The model under review builds one solid part; all positions refer to its coordinate system, in mm. Face numbers are marked on the shaded views. A direction names the side the tool comes from. Give positions to 0.01 mm unless a question says otherwise; leave off trailing zeros. Order: outer loops, then holes, each group sorted by start corner. A loop starts at its lowest first (then second) coordinate and runs counter-clockwise, first axis right, second up. Notation, with made-up numbers: (10, 63) - (59, 63) arc R17 cw to (59, 94) - close; hole circle Ø5 at (25, -12). An arc over 180 degrees is marked (long way). Use CSV: the item, a comma, the result in double quotes.
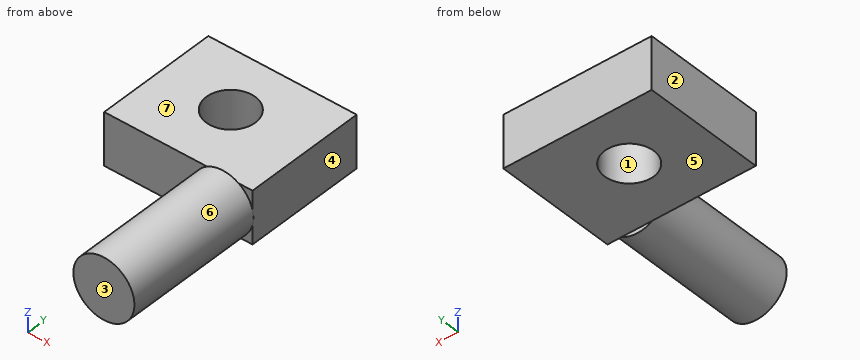
Autodesk Inventor part; units mm, degrees
ref_plane "YZ Plane" through (0, 0, 0) normal (1, 0, 0) x (0, 1, 0)
ref_plane "XZ Plane" through (0, 0, 0) normal (0, 1, 0) x (-1, 0, 0)
ref_plane "XY Plane" through (0, 0, 0) normal (0, 0, 1) x (1, 0, 0)
sketch "Sketch1" plane through (0, 0, 0) normal (0, 1, 0) x (-1, 0, 0)
  circle A0 centre (0, 0) radius 17.5
  dimension "d0" = 35
extrude "Extrusion1" add sketch "Sketch1" along normal blind 80
sketch "Sketch2" plane through (0, 80, 0) normal (0, 1, 0) x (1, 0, 0)
  line L0 (-68, -15) -> (17, -15)
  line L1 (17, -15) -> (17, 15)
  line L2 (17, 15) -> (-68, 15)
  line L3 (-68, 15) -> (-68, -15)
  point P0 (0, 0)
  dimension "d3" = 85
  dimension "d4" = 30
extrude "Extrusion2" add sketch "Sketch2" along normal blind 70
sketch "Sketch3" plane through (-68, 80, 15) normal (0, 0, 1) x (1, 0, 0)
  circle A0 centre (41, 37) radius 14
  point P0 (68, -80)
extrude "Extrusion3" cut sketch "Sketch3" against normal through all
properties part number "motor hombro"
Item 1: Wall thickness on L1, parallel to Y at x = -27, z = 6; L2, parallel to Z at x = -60.5, y = 123; L3, parallel to Y at x = -48, z = -2.5: over which ranges is each line inside the solid? List them lowest first.
Results list:
L1,"y = 80 to 103, 131 to 150"
L2,"z = -15 to 15"
L3,"y = 80 to 150"
Item 2: Take a section at B-B, the plane z = 0. Give the boundary of the cut face in (x, y), and give its area (3 significant figures).
Results list:
outline,"(-68, 80) - (-17.5, 80) - (-17.5, 0) - (17.5, 0) - (17.5, 80) - (17, 80) - (17, 150) - (-68, 150) - close; hole circle Ø28 at (-27, 117)"
area,"8,130 mm2"
Item 3: Mouldability with a two-part tool opening along X and no side actions: class the marked faces 1, 2, 3 and 4 as pulls with the +X half, pulls with the -X half, needs draft (parallel to the pull), parting line crosses it, or undercut.
Results list:
face 1,"undercut"
face 2,"pulls with the -X half"
face 3,"needs draft"
face 4,"pulls with the +X half"
Item 4: Take a section at C-C, the plane x = -31. Give the boundary of the cut face in (y, z).
Results list:
outline,"(80, -15) - (103.58, -15) - (103.58, 15) - (80, 15) - close; (130.42, -15) - (150, -15) - (150, 15) - (130.42, 15) - close"
Item 5: Take a section at D-D, the plane x = 0. Give the boundary of the cut face in (y, z), and give its area (3 significant figures).
Results list:
outline,"(0, -17.5) - (80, -17.5) - (80, -15) - (150, -15) - (150, 15) - (80, 15) - (80, 17.5) - (0, 17.5) - close"
area,"4,900 mm2"
Item 6: Clearance check with flat-ended pins moving along their axes: pin 1 (9 mm diameter, centred on x = -33, z = -4, fed in from -Y); pin 2 (8 mm diameter, centred on y = 40, z = -10.5, fed in from -X); pin 3 (6 mm diameter, centred on y = 103, z = 13, fed in from +X); pin 4 (22.5 mm diameter, centred on x = -27, y = 117, fed in from +Z). State where each tip first meets the part, or that it passes through.
Results list:
pin 1,"stops at y = 80"
pin 2,"stops at x = -16.25"
pin 3,"stops at x = 17"
pin 4,"passes through"
Item 7: Take a section at A-A, the plane y = 117. Give the boundary of the cut face in (x, z), and give its area (3 significant figures).
Results list:
outline,"(-68, -15) - (-41, -15) - (-41, 15) - (-68, 15) - close; (-13, -15) - (17, -15) - (17, 15) - (-13, 15) - close"
area,"1,710 mm2"
Item 8: Tool access review of the marked faces 5, 6 and 7: name each direction out of +Z, -Z, +X, -X, +Y, -Y from which nothing blocks a thin tool from reaching the whole face with its end or side.
Results list:
face 5,"-Z, +X, -X, +Y"
face 6,"-Y"
face 7,"+Z, +X, -X, +Y"
